```python
from build123d import *

# Parameters (mm, degrees)
SKETCH1_W           = 7.5
SKETCH1_H           = 20
BOSS_EXTRUDE2_DEPTH = 2
SKETCH2_W           = 7.5
SKETCH2_H           = 1.98347932
BOSS_EXTRUDE3_DEPTH = 20
SKETCH3_W           = 7.5
SKETCH3_H           = 2
BOSS_EXTRUDE4_DEPTH = 20
SKETCH5_R           = 1.5
CUT_EXTRUDE1_DEPTH  = 20
SKETCH7_W           = 20
SKETCH7_H           = 2
BOSS_EXTRUDE6_DEPTH = 6
SKETCH8_W           = 20
SKETCH8_H           = 1.98347932
BOSS_EXTRUDE7_DEPTH = 6
SKETCH9_R           = 1.75
CUT_EXTRUDE2_DEPTH  = 6


with BuildPart() as part:
    # Sketch1 → Boss-Extrude2 (new body)
    with BuildSketch(Plane(origin=(0, 0, 0), x_dir=(0, 0, -1), z_dir=(1, 0, 0))):
        with Locations((3.009581882, -0.975609756)):
            Rectangle(SKETCH1_W, SKETCH1_H)
    extrude(amount=BOSS_EXTRUDE2_DEPTH)

    # Sketch2 → Boss-Extrude3 (add)
    with BuildSketch(Plane(origin=(2, 0, 0), x_dir=(0, 0, -1), z_dir=(1, 0, 0))):
        with Locations((3.009581882, -9.983870096)):
            Rectangle(SKETCH2_W, SKETCH2_H)
    extrude(amount=BOSS_EXTRUDE3_DEPTH)

    # Sketch3 → Boss-Extrude4 (add)
    with BuildSketch(Plane(origin=(2, 0, 0), x_dir=(0, 0, -1), z_dir=(1, 0, 0))):
        with Locations((3.009581882, -6.242130436)):
            Rectangle(SKETCH3_W, SKETCH3_H)
    extrude(amount=BOSS_EXTRUDE4_DEPTH)

    # Sketch5 → Cut-Extrude1 (cut)
    with BuildSketch(Plane(origin=(2, 0, 0), x_dir=(0, 0, -1), z_dir=(1, 0, 0))):
        with Locations((3.009581882, 5.024390244)):
            Circle(SKETCH5_R)
        with Locations((3.096458319, -1.242130436)):
            Circle(SKETCH5_R)
    extrude(amount=-CUT_EXTRUDE1_DEPTH, mode=Mode.SUBTRACT)

    # Sketch7 → Boss-Extrude6 (add)
    with BuildSketch(Plane(origin=(0, 0, -6.759581882), x_dir=(-1, 0, 0), z_dir=(0, 0, -1))):
        with Locations((-12, -6.242130436)):
            Rectangle(SKETCH7_W, SKETCH7_H)
    extrude(amount=BOSS_EXTRUDE6_DEPTH)

    # Sketch8 → Boss-Extrude7 (add)
    with BuildSketch(Plane(origin=(0, 0, -6.759581882), x_dir=(-1, 0, 0), z_dir=(0, 0, -1))):
        with Locations((-12, -9.983870096)):
            Rectangle(SKETCH8_W, SKETCH8_H)
    extrude(amount=BOSS_EXTRUDE7_DEPTH)

    # Sketch9 → Cut-Extrude2 (cut)
    with BuildSketch(Plane(origin=(0, -5.242130436, 0), x_dir=(1, 0, 0), z_dir=(0, 1, 0))):
        with Locations((10, 8.759581882)):
            Circle(SKETCH9_R)
    extrude(amount=-CUT_EXTRUDE2_DEPTH, mode=Mode.SUBTRACT)


solid = part.part
```
The model under review builds one solid part; all positions refer to its coordinate system, in mm. A direction names the side the tool comes from. Round coordinates to 2 decimals unless told otherwise and drop trailing zeros. Order: outer loops, then holes, each group sorted by start corner. A loop starts at its lowest first (then second) coordinate and runs counter-clockwise, first axis right, second up. Notation, with made-up numbers: (2, 38) -> (9, 38) arc R32 cw to (9, 65) -> close; hole circle Ø6 at (48, 9.5). An arc over 180 degrees is marked (long way). One line per item, written item: value. Start each with the question number.
Q1. Take a section at D-D (y = -5.75). Write out the cut boundary in (x, z).
Q2. Clearance check with flat-ended pins moving along their axes: pin 1 Ø12 at (x, y) = (3, -0.5) entering from -Z; pin 2 Ø2 at (y, z) = (-10, -8.5) entering from -X; pin 3 Ø8 at (y, z) = (3, -2.5) entering from +X; pin 4 Ø7 at (x, z) = (9, -5) entering from +Y. State where each tip first meets the part, or that it passes through.
Q3. Take a section at B-B (z = -10). Write out the cut boundary in (x, y), and give its area (3 significant figures).
Q4. Machinability: for faces 4 (the face through (1, -1, -6.76)), 5 (the face through (12, -8.992, -6)), 6 (the face through (12, -5.242, -6)), which of the approach directions +Z, -Z, +X, -X, +Y, -Y give a long, thin tool a straight path to every point of the face, cutting with its end or side? Answer none if there is none.
Q5. Take a section at A-A (x = 17.5). Write out the cut boundary in (y, z).
Q6. Mouldability with a two-part tool opening along X and no side actions: class faces 1 (the face through (2, -10, -10)), 2 (the face through (10.81, -9.97, -7.21)), 3 (the face through (11, -10.976, -6)) as released by +X, released by -X, zero draft, split by the parting line, or undercut.
Q7. Wall thickness on line 1 (Y direction, x = 9.5, z = -0.25); line 2 (Z direction, x = 10, y = -9.6); line 3 (X direction, y = 2.75, z = -5): over which ranges is each line inside the solid? List them lowest first.
Q8. Take a section at C-C (x = 10). Write out the cut boundary in (y, z).
Reported:
1. outline: (0, -6.76) -> (2, -6.76) -> (2, -12.76) -> (22, -12.76) -> (22, 0.74) -> (0, 0.74) -> close; hole circle Ø3.5 at (10, -8.76)
2. pin 1: stops at z = -12.76
2. pin 2: stops at x = 2
2. pin 3: stops at x = 2
2. pin 4: stops at y = -5.24
3. outline: (2, -10.98) -> (8.77, -10.98) -> (8.77, -8.99) -> (2, -8.99) -> close; (2, -7.24) -> (8.77, -7.24) -> (8.77, -5.24) -> (2, -5.24) -> close; (11.23, -10.98) -> (22, -10.98) -> (22, -8.99) -> (11.23, -8.99) -> close; (11.23, -7.24) -> (22, -7.24) -> (22, -5.24) -> (11.23, -5.24) -> close
3. area: 69.8 mm2
4. face 4: -Z, -X, +Y, -Y
4. face 5: +Z, -Z, +X
4. face 6: +Z, -Z, +X, +Y
5. outline: (-10.98, -12.76) -> (-8.99, -12.76) -> (-8.99, 0.74) -> (-10.98, 0.74) -> close; (-7.24, -12.76) -> (-5.24, -12.76) -> (-5.24, 0.74) -> (-7.24, 0.74) -> close
6. face 1: released by -X
6. face 2: undercut
6. face 3: zero draft
7. line 1: y = -10.98 to -8.99, -7.24 to -5.24
7. line 2: z = -12.76 to -10.51, -7.01 to 0.74
7. line 3: x = 0 to 2
8. outline: (-10.98, -12.76) -> (-8.99, -12.76) -> (-8.99, -10.51) -> (-10.98, -10.51) -> close; (-10.98, -7.01) -> (-8.99, -7.01) -> (-8.99, 0.74) -> (-10.98, 0.74) -> close; (-7.24, -12.76) -> (-5.24, -12.76) -> (-5.24, -10.51) -> (-7.24, -10.51) -> close; (-7.24, -7.01) -> (-5.24, -7.01) -> (-5.24, 0.74) -> (-7.24, 0.74) -> close
